Work out the finished part from the listing and answer in its coordinate system (mm). Face numbers are marked on the shaded views. A direction names the side the tool comes from. Coordinates: 2 decimals unless noted, no trailing zeros. Loops run counter-clockwise (first coordinate to the right, second up) from the corner with the lowest first, then second, coordinate; pieces in that order, holes last. Notation, with made-up numbers: (22, 16) -> (38, 16) arc R35 cw to (38, 51) -> close; hole circle Ø9 at (29, 1.25). An arc over 180 degrees is marked (long way). Answer as CSV lines item,"result".
```python
from build123d import *

# Parameters (mm, degrees)
BOSS_EXTRUDE1_DEPTH = 12
SKETCH2_W           = 30
SKETCH2_H           = 2.5
CUT_EXTRUDE1_DEPTH  = 10
FILLET1_R           = 10
FILLET2_R           = 4
SKETCH5_W           = 57.951370105
SKETCH5_H           = 2.5
CUT_EXTRUDE2_DEPTH  = 43.617484675
FILLET3_R           = 1
FILLET4_R           = 1
SKETCH6_R           = 3
SKETCH6_R_2         = 2.5
BOSS_EXTRUDE2_DEPTH = 1


with BuildPart() as part:
    # Sketch1 → Boss-Extrude1 (new body)
    with BuildSketch(Plane(origin=(0, 0, 0), x_dir=(1, 0, 0), z_dir=(0, 1, 0))):
        Polygon((10, 0), (1.5, 0), (1.5, 40), (5, 10), (10, 10), align=None)
    extrude(amount=BOSS_EXTRUDE1_DEPTH)

    # Sketch2 → Cut-Extrude1 (cut)
    with BuildSketch(Plane.ZY.offset(-1.5)):
        with Locations((-25, 1.25)):
            Rectangle(SKETCH2_W, SKETCH2_H)
    extrude(amount=-CUT_EXTRUDE1_DEPTH, mode=Mode.SUBTRACT)

    # Fillet1
    # the kernel refuses this fillet: 10 mm, written as the material it adds along each edge
    with BuildSketch(Plane(origin=(5, 2.5, -10), x_dir=(1, 0, 0), z_dir=(0, 1, 0))) as fillet1_piece_1:
        with BuildLine():
            CenterArc((8.998480528, 9.165814392), FILLET1_R, 186.654425046, 59.776895084)
            Line((-0.934150863, 8.007007396), (-1.132803491, 7.983831256))
            Line((-1.132803491, 7.983831256), (-0.198652628, -0.02317614))
            Line((-0.198652628, -0.02317614), (0, -0.2))
            ThreePointArc((0, -0.2), (2.5, -0.2), (4.920030389, -0.183316288))
            Line((4.920030389, -0.183316288), (5, 0))
        make_face()
    extrude(amount=9.5)

    # Fillet2
    fillet2_edges = [part.edges().sort_by_distance(p)[0] for p in [
        (1.5, 6, 0),
    ]]
    fillet(fillet2_edges, radius=FILLET2_R)

    # Sketch5 → Cut-Extrude2 (cut, through all)
    with BuildSketch(Plane(origin=(10, 0, 0), x_dir=(0, 0, -1), z_dir=(1, 0, 0))):
        with Locations((38.975685053, 10.75)):
            Rectangle(SKETCH5_W, SKETCH5_H)
    extrude(amount=-CUT_EXTRUDE2_DEPTH, mode=Mode.SUBTRACT)

    # Fillet3
    # the kernel refuses this fillet: 1 mm, written as the material it adds along each edge
    with BuildSketch(Plane(origin=(10, 9.5, -10), x_dir=(0, 1, 0), z_dir=(-1, 0, 0))) as fillet3_piece_1_section:
        with BuildLine():
            CenterArc((FILLET3_R, FILLET3_R), FILLET3_R, 180, 90)
            Line((0, FILLET3_R), (0, 0))
            Line((0, 0), (FILLET3_R, 0))
        make_face()
    fillet3_piece_1 = extrude(amount=8.5, mode=Mode.PRIVATE)
    fillet3_piece_1 = fillet3_piece_1 - Plane(origin=(13.998480528, 9.732981391, -19.165814392), x_dir=(1, 0, 0), z_dir=(0, -1, 0)) * Cylinder(10, 22, mode=Mode.PRIVATE)
    add(fillet3_piece_1)

    # Fillet4
    # the kernel refuses this fillet: 1 mm, written as the material it adds along each edge
    with BuildSketch(Plane(origin=(10, 2.5, -10), x_dir=(0, 0, -1), z_dir=(-1, 0, 0))) as fillet4_piece_1_section:
        with BuildLine():
            CenterArc((FILLET4_R, FILLET4_R), FILLET4_R, 180, 90)
            Line((0, FILLET4_R), (0, 0))
            Line((0, 0), (FILLET4_R, 0))
        make_face()
    fillet4_piece_1 = extrude(amount=8.5, mode=Mode.PRIVATE)
    fillet4_piece_1 = fillet4_piece_1 - Plane(origin=(13.998480528, 2.267019068, -19.165814392), x_dir=(1, 0, 0), z_dir=(0, -1, 0)) * Cylinder(10, 21, mode=Mode.PRIVATE)
    add(fillet4_piece_1)

    # Sketch6 → Boss-Extrude2 (add)
    with BuildSketch(Plane(origin=(10, 0, 0), x_dir=(0, 0, -1), z_dir=(1, 0, 0))):
        with Locations((5, 6)):
            Circle(SKETCH6_R)
        with Locations((5, 6)):
            Circle(SKETCH6_R_2, mode=Mode.SUBTRACT)
    extrude(amount=BOSS_EXTRUDE2_DEPTH)


solid = part.part
```
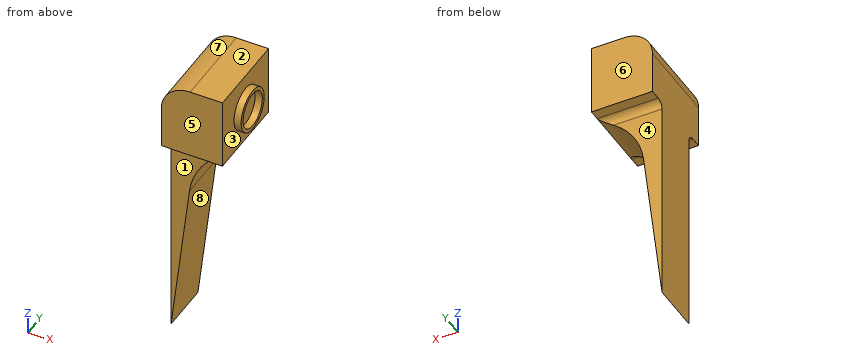
(1) A cutting plane is placed at C-C, the plane y = 8. Write down the section's boundary in (x, z).
Computed values:
outline,"(1.5, -40) -> (4.07, -18.01) arc R10 cw to (10, -10) -> (10, -7.24) -> (11, -7.24) -> (11, -6.5) -> (10, -6.5) -> (10, -3.5) -> (11, -3.5) -> (11, -2.76) -> (10, -2.76) -> (10, 0) -> (5.5, 0) arc R4 ccw to (1.5, -4) -> close"
(2) A cutting plane is placed at A-A, the plane y = 6. Write down the section's boundary in (x, z).
Computed values:
outline,"(1.5, -40) -> (4.07, -18.01) arc R10 cw to (10, -10) -> (10, -8) -> (11, -8) -> (11, -7.5) -> (10, -7.5) -> (10, -2.5) -> (11, -2.5) -> (11, -2) -> (10, -2) -> (10, 0) -> (5.5, 0) arc R4 ccw to (1.5, -4) -> close"
(3) A cutting plane is placed at D-D, the plane z = -22.5. Write down the section's boundary in (x, y), and give its area (3 significant figures).
Computed values:
outline,"(1.5, 2.5) -> (3.54, 2.5) -> (3.54, 9.5) -> (1.5, 9.5) -> close"
area,"14.3 mm2"
(4) A cutting plane is placed at B-B, the plane z = -5. Write down the section's boundary in (x, y), and give its area (3 significant figures).
Computed values:
outline,"(1.5, 0) -> (10, 0) -> (10, 3) -> (11, 3) -> (11, 3.5) -> (10, 3.5) -> (10, 8.5) -> (11, 8.5) -> (11, 9) -> (10, 9) -> (10, 12) -> (1.5, 12) -> close"
area,"103 mm2"
(5) For a pull along Z with two mould halves and no side action, classify the marked faces 6, 7 and 8 as pulls with the +Z half, pulls with the -Z half, needs draft (parallel to the pull), parting line crosses it, or undercut.
Computed values:
face 6,"needs draft"
face 7,"pulls with the +Z half"
face 8,"pulls with the -Z half"
(6) Which of the six approach directions +Z, -Z, +X, -X, +Y, -Y give full straight-line access (tool end or side, diameter ignored) to the marked faces 1, 2, 3, 4 and 5?
Computed values:
face 1,"-Z, +X, -X, -Y"
face 2,"+Z, +X, -X, +Y, -Y"
face 3,"+X"
face 4,"-Z, +X, -X, +Y"
face 5,"+Z, -Z, +X, -X, -Y"
(7) Flat-ended cylindrical pins translate along their axes: pin 1 Ø1.5 at (y, z) = (5.5, -4) entering from +X; pin 2 Ø6.5 at (y, z) = (6, -5) entering from +X; pin 3 Ø2 at (x, z) = (3, -18) entering from -Y; pin 4 Ø2 at (x, z) = (6, -21.5) entering from +Y. Find the tip coordinate at first contact, or state that the pin passes through.
Computed values:
pin 1,"x = 10"
pin 2,"x = 11"
pin 3,"y = 2.5"
pin 4,"through"
(8) Consider line 1 along Y through (x, z) = (10.3, -5); line 2 along X through (y, z) = (2.25, -9.5); line 3 along Y through (x, z) = (4, -13.5). Determine where each line is inside the solid, lowest interval first.
Computed values:
line 1,"3 to 3.5, 8.5 to 9"
line 2,"1.5 to 10"
line 3,"2.5 to 9.5"
